The model under review builds one solid part; all positions refer to its coordinate system, in mm. Face numbers are marked on the shaded views. A direction names the side the tool comes from. Give positions to 0.01 mm unless a question says otherwise; leave off trailing zeros. Order: outer loops, then holes, each group sorted by start corner. A loop starts at its lowest first (then second) coordinate and runs counter-clockwise, first axis right, second up. Notation, with made-up numbers: (-15.5, 51.25) -> (13.5, 51.25) arc R24 cw to (13.5, 81.25) -> close; hole circle Ø10 at (-21.75, -8.75). An arc over 180 degrees is marked (long way). Use one line per item in the form item = value.
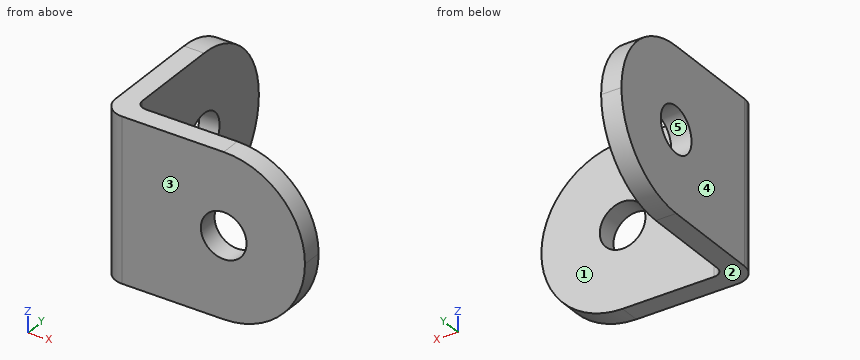
```python
from build123d import *

# Parameters (mm, degrees)
EXTRUDE_1_DEPTH     = 16
CUT_EXTRUDE_1_DEPTH = 21
CUT_EXTRUDE_2_DEPTH = 21
FILLET_1_R          = 1
FILLET_2_R          = 2
SKETCH_4_R          = 2.25
CUT_EXTRUDE_3_DEPTH = 3
SKETCH_5_R          = 2.25
CUT_EXTRUDE_4_DEPTH = 3


with BuildPart() as part:
    # Sketch 1 → Бобышка-Вытянуть1 (new body)
    with BuildSketch(Plane.XY):
        Polygon((0, 0), (0, 20), (2, 20), (2, 2), (20, 2), (20, 0), align=None)
    extrude(amount=EXTRUDE_1_DEPTH)

    # Эскиз2 → Вырез-Вытянуть1 (cut, through all)
    with BuildSketch(Plane.XZ):
        with BuildLine():
            Line((20, 0), (20, 8.000000031))
            ThreePointArc((20, 8.000000031), (17.656854261, 2.343145762), (12, 0))
            Line((12, 0), (20, 0))
        make_face()
        with BuildLine():
            Line((20, 16), (12, 16))
            ThreePointArc((12, 16), (17.656854238, 13.656854261), (20, 8.000000031))
            Line((20, 8.000000031), (20, 16))
        make_face()
    extrude(amount=-CUT_EXTRUDE_1_DEPTH, mode=Mode.SUBTRACT)

    # Эскиз3 → Вырез-Вытянуть2 (cut, through all)
    with BuildSketch(Plane.ZY):
        with BuildLine():
            Line((8, 20), (0, 20))
            Line((0, 20), (0, 12))
            ThreePointArc((0, 12), (2.343145751, 17.656854249), (8, 20))
        make_face()
        with BuildLine():
            Line((16, 20), (8, 20))
            ThreePointArc((8, 20), (13.656854249, 17.656854249), (16, 12))
            Line((16, 12), (16, 20))
        make_face()
    extrude(amount=-CUT_EXTRUDE_2_DEPTH, mode=Mode.SUBTRACT)

    # Скругление1
    fillet_1_edges = [part.edges().sort_by_distance(p)[0] for p in [
        (2, 2, 8),
    ]]
    fillet(fillet_1_edges, radius=FILLET_1_R)

    # Скругление2
    fillet_2_edges = [part.edges().sort_by_distance(p)[0] for p in [
        (0, 0, 8),
    ]]
    fillet(fillet_2_edges, radius=FILLET_2_R)

    # Эскиз4 → Вырез-Вытянуть3 (cut, through all)
    with BuildSketch(Plane(origin=(2, 0, 0), x_dir=(0, 0, -1), z_dir=(1, 0, 0))):
        with Locations((-8, 12)):
            Circle(SKETCH_4_R)
    extrude(amount=-CUT_EXTRUDE_3_DEPTH, mode=Mode.SUBTRACT)

    # Эскиз5 → Вырез-Вытянуть4 (cut, through all)
    with BuildSketch(Plane(origin=(0, 2, 0), x_dir=(1, 0, 0), z_dir=(0, 1, 0))):
        with Locations((12, -8)):
            Circle(SKETCH_5_R)
    extrude(amount=-CUT_EXTRUDE_4_DEPTH, mode=Mode.SUBTRACT)


solid = part.part
```
1. Tool access review of the marked faces 1 and 2: name each direction out of +Z, -Z, +X, -X, +Y, -Y from which nothing blocks a thin tool from reaching the whole face with its end or side.
Values:
face_1 = +Z, -Z, +X, +Y
face_2 = -Z, +X, -X, +Y, -Y
2. Add section D-D on z = 12. Give the boundary of the cut face in (x, y), then the cut area to 3 significant figures.
Values:
outline = (0, 2) arc R2 ccw to (2, 0) -> (18.93, 0) -> (18.93, 2) -> (3, 2) arc R1 cw to (2, 3) -> (2, 18.93) -> (0, 18.93) -> close
area = 71.1 mm^2
3. Add section B-B on z = 3.5. Give the boundary of the cut face in (x, y).
Values:
outline = (0, 2) arc R2 ccw to (2, 0) -> (18.61, 0) -> (18.61, 2) -> (3, 2) arc R1 cw to (2, 3) -> (2, 18.61) -> (0, 18.61) -> close
4. For pin 1 Ø6 at (y, z) = (7.5, 2) entering from +X; pin 2 Ø1.5 at (x, z) = (3, 14.5) entering from +Y; pin 3 Ø5 at (x, z) = (13.5, 5.5) entering from +Y, all flat-tipped, find the tip position at first contact; note any pin that passes through.
Values:
pin_1 = 2
pin_2 = 2.34
pin_3 = 2
5. Add section C-C on x = 3.5. Give the boundary of the cut face in (y, z), then the cut area to 3 significant figures.
Values:
outline = (0, 0) -> (2, 0) -> (2, 16) -> (0, 16) -> close
area = 32.0 mm^2
6. Add section A-A on y = 10.75. Give the boundary of the cut face in (x, z), then the cut area to 3 significant figures.
Values:
outline = (0, 0) -> (2, 0) -> (2, 6.13) -> (0, 6.13) -> close; (0, 9.87) -> (2, 9.87) -> (2, 16) -> (0, 16) -> close
area = 24.5 mm^2
7. The part is to be moulded in two halves that separate along Y. For the marked faces 3, 4 and 5, say which applies: +Y half, -Y half, draft (parallel to the pull), parting line (faces both ways), or undercut.
Values:
face_3 = -Y half
face_4 = draft
face_5 = undercut
8. For L1, parallel to Z at x = 12, y = 1.1; L2, parallel to X at y = 4.5, z = 1.5, list the stretches that pass through material, from the lowest coordinate up.
Values:
L1 = 0 to 5.75, 10.25 to 16
L2 = 0 to 2
